from build123d import *

# Parameters (mm, degrees)
F1_DEPTH     = 43
F2_W         = 20
F2_H         = 20
F3_DEPTH     = 3
F4_W         = 27
F4_H         = 20
F5_DEPTH     = 5
F7_R         = 12.5
F8_DEPTH     = 5
F11_D        = 3.2
F11_ON_F9_D  = 3.2
F11_ON_F10_D = 3.2
F12_W        = 21
F12_H        = 20
F13_DEPTH    = 5
F14_SIZE     = 20
F15_R        = 2.5
F16_DEPTH    = 8


with BuildPart() as f1:
    # F0 (on Front) → F1 (new body)
    with BuildSketch(Plane.XZ):
        Polygon((0, 25), (0, 20), (20, 20), (20, 0), (25, 0), (25, 20), (46, 20), (46, 25), (24, 25), (24, 68), (19, 68), (19, 25), align=None)
    extrude(amount=F1_DEPTH)

    # F2 (on face) → F3 (join)
    with BuildSketch(Plane.XZ.offset(43)):
        with Locations((10, 10)):
            Rectangle(F2_W, F2_H)
    extrude(amount=-F3_DEPTH)

    # F4 (on face) → F5 (cut, through all)
    with BuildSketch(Plane.YZ.offset(25)):
        with Locations((-13.5, 10)):
            Rectangle(F4_W, F4_H)
    extrude(amount=-F5_DEPTH, mode=Mode.SUBTRACT)

    # F7 (on face) → F8 (cut, through all)
    with BuildSketch(Plane.YZ.offset(24)):
        with Locations((-21.5, 46.5)):
            Circle(F7_R)
    extrude(amount=-F8_DEPTH, mode=Mode.SUBTRACT)

    # F11 (through all)
    with Locations(Plane.YZ.offset(24)):
        with Locations((-37, 62), (-6, 62), (-37, 31), (-6, 31)):
            Hole(F11_D / 2)

    # F11 on F9 (through all)
    with Locations(Plane(origin=(0, 0, 20), x_dir=(1, 0, 0), z_dir=(0, 0, -1))):
        with Locations((10, 10), (10, 30)):
            Hole(F11_ON_F9_D / 2)

    # F11 on F10 (through all)
    with Locations(Plane(origin=(20, 0, 0), x_dir=(0, -1, 0), z_dir=(-1, 0, 0))):
        with Locations((33.5, 10)):
            Hole(F11_ON_F10_D / 2)

    # F12 (on face) → F13 (join)
    with BuildSketch(Plane.XZ.offset(43)):
        Polygon((19, 68), (0, 25), (19, 25), align=None)
        Polygon((19, 25), (0, 25), (0, 0), (25, 0), (25, 20), (46, 20), (46, 25), (24, 25), (24, 68), (19, 68), align=None)
        Polygon((46, 25), (24, 68), (24, 25), align=None)
        with Locations((35.5, 10)):
            Rectangle(F12_W, F12_H)
    extrude(amount=F13_DEPTH)

    # F14
    f14_edges = [f1.edges().sort_by_distance(p)[0] for p in [
        (46, 0, 22.5),
    ]]
    chamfer(f14_edges, length=F14_SIZE)

    # F15 (on face) → F16 (cut, through all)
    with BuildSketch(Plane(origin=(0, -40, 0), x_dir=(-1, 0, 0), z_dir=(0, 1, 0))):
        with Locations((-10, 10)):
            Circle(F15_R)
    extrude(amount=-F16_DEPTH, mode=Mode.SUBTRACT)


solid = f1.part
The model under review builds one solid part; all positions refer to its coordinate system, in mm. A direction names the side the tool comes from. Round coordinates to 2 decimals unless told otherwise and drop trailing zeros. Order: outer loops, then holes, each group sorted by start corner. A loop starts at its lowest first (then second) coordinate and runs counter-clockwise, first axis right, second up. Notation, with made-up numbers: (-36, 73) -> (-11, 73) arc R30 ccw to (-11, 112) -> close; hole circle Ø7 at (15.5, 55). An arc over 180 degrees is marked (long way). Use CSV: the item, a comma, the result in double quotes. Start each with the question number.
(1) Consider section D-D on x = 23. Write out the cut boundary in (y, z), and give its area (3 significant figures).
(2) Insertion check: pin 1 (13 mm diameter, centred on y = -27, z = 42, fed in from +X); pin 2 (3 mm diameter, centred on x = 10, z = 10, fed in from -Y); pin 3 (1 mm diameter, centred on x = 18, y = -27, fed in from -Z); pin 4 (15 mm diameter, centred on x = 11, y = -13, fed in from +Z). Each pin has a flat end and moves straight along its axis. Give the tip position at first contact, or say it passes through.
(3) Mouldability with a two-part tool opening along Y and no side actions: class faces 4 (the face through (21.47, -6.74, 29.58)), 5 (the face through (25, -37, 10)), 6 (the face through (35, -43, 10)) as pulls with the +Y half, pulls with the -Y half, needs draft (parallel to the pull), parting line crosses it, or undercut.
(4) Wall thickness on probe 1 along Z at (x, y) = (20.45, -37); probe 2 along X at (y, z) = (-17, 29); probe 3 along Z at (x, y) = (26, -32.5): over which ranges is each line inside the solid? List them lowest first. Write a range as from..to.
(5) Consider section B-B on z = 23. Write out the cut boundary in (x, y), and give its area (3 significant figures).
(6) Tool access review of faces 1 (the face through (22, -24, 68)), 2 (the face through (24, -31, 56)), 3 (the face through (10, -21, 25)): name each direction out of +Z, -Z, +X, -X, +Y, -Y from which nothing blocks a thin tool from reaching the whole face with its end or side.
(7) Consider section C-C on y = -21.5. Write out the cut boundary in (x, z), and give its area (3 significant figures).
(8) Consider section A-A on y = -6. Write out the cut boundary in (x, z).
Responses:
1,outline,"(-48, 0) -> (-27, 0) -> (-27, 20) -> (0, 20) -> (0, 68) -> (-48, 68) -> close; hole circle Ø3.2 at (-37, 31); hole circle Ø3.2 at (-37, 62); hole circle Ø3.2 at (-33.5, 10); hole circle Ø25 at (-21.5, 46.5); hole circle Ø3.2 at (-6, 31); hole circle Ø3.2 at (-6, 62)"
1,area,"2,190 mm²"
2,pin 1,"x = 24"
2,pin 2,"through"
2,pin 3,"z = 20"
2,pin 4,"z = 25"
3,face 4,"undercut"
3,face 5,"needs draft"
3,face 6,"pulls with the +Y half"
4,probe 1,"0..29.4, 32.6..60.4, 63.6..68"
4,probe 2,"19..24"
4,probe 3,"20..25"
5,outline,"(0, -48) -> (46, -48) -> (46, -20) -> (26, 0) -> (0, 0) -> close; hole circle Ø3.2 at (10, -30); hole circle Ø3.2 at (10, -10)"
5,area,"1,990 mm²"
6,face 1,"+Z, +X, -X, +Y, -Y"
6,face 2,"+Z, +X, +Y"
6,face 3,"+Z, -X, +Y"
7,outline,"(0, 20) -> (46, 20) -> (46, 25) -> (24, 25) -> (24, 34) -> (19, 34) -> (19, 25) -> (0, 25) -> close; (19, 59) -> (24, 59) -> (24, 68) -> (19, 68) -> close"
7,area,"320 mm²"
8,outline,"(0, 20) -> (32, 20) -> (32, 25) -> (24, 25) -> (24, 29.4) -> (19, 29.4) -> (19, 25) -> (0, 25) -> close; (19, 32.6) -> (24, 32.6) -> (24, 60.4) -> (19, 60.4) -> close; (19, 63.6) -> (24, 63.6) -> (24, 68) -> (19, 68) -> close"
